Study the drawing (mm; zero at the part's minimum x, y, z) and answer. A direction names the side the tool comes from. Give positions to 0.01 mm unless a question says otherwise; leave off trailing zeros. Order: outer loops, then holes, each group sorted by start corner. A loop starts at its lowest first (then second) coordinate and runs counter-clockwise, first axis right, second up. Notation, with made-up numbers: (-21, 73) - (16, 73) arc R30 cw to (16, 104) - close; hole circle Ø3 at (-25, 48.25). An arc over 180 degrees is marked (long way). Return JSON: item names as keys, results as strings.
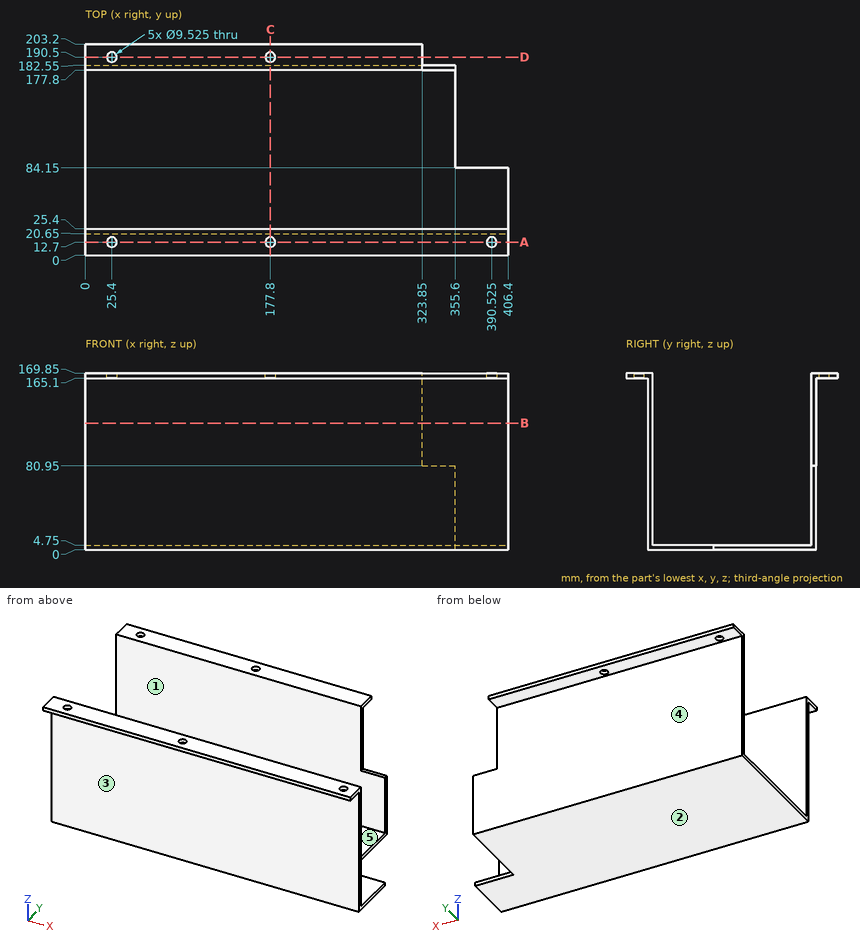
Q1. Given pin 1 (4 mm diameter, centred on x = 268, z = 87.5, fed in from -Y); pin 2 (8.5 mm diameter, centred on x = 25.4, y = 190.5, fed in from -Z); pin 3 (1.4 mm diameter, centred on x = 379.5, z = 1, fed in from +Y); pin 4 (10.5 mm diameter, centred on x = 215.5, y = 10, fed in from -Z), each flat-ended and moving along its own axis, determine where each tip first touches the part or whether it passes through.
Values:
{"pin 1": "stops at y = 20.65", "pin 2": "passes through", "pin 3": "stops at y = 84.15", "pin 4": "stops at z = 165.1"}
Q2. For the marked faces 4 and 5, determine the directions among +Z, -Z, +X, -X, +Y, -Y from which every point of the face is accessible in a straight line to the end or side of a thin tool.
Values:
{"face 4": "-Z, +X, -X, +Y", "face 5": "+Z, +X, -X"}
Q3. A cutting plane is placed at A-A (y = 12.7). Write down the section's boundary in (x, z).
Values:
{"outline": "(0, 165.1) - (20.64, 165.1) - (20.64, 169.85) - (0, 169.85) - close; (30.16, 165.1) - (173.04, 165.1) - (173.04, 169.85) - (30.16, 169.85) - close; (182.56, 165.1) - (385.76, 165.1) - (385.76, 169.85) - (182.56, 169.85) - close; (395.29, 165.1) - (406.4, 165.1) - (406.4, 169.85) - (395.29, 169.85) - close"}
Q4. A cutting plane is placed at D-D (y = 190.5). Write down the section's boundary in (x, z).
Values:
{"outline": "(0, 165.1) - (20.64, 165.1) - (20.64, 169.85) - (0, 169.85) - close; (30.16, 165.1) - (173.04, 165.1) - (173.04, 169.85) - (30.16, 169.85) - close; (182.56, 165.1) - (323.85, 165.1) - (323.85, 169.85) - (182.56, 169.85) - close"}
Q5. Determine the mould class of the marked faces 1, 2 and 3 for opening direction Y: released by +Y, released by -Y, zero draft, split by the parting line, or undercut.
Values:
{"face 1": "undercut", "face 2": "zero draft", "face 3": "released by -Y"}
Q6. Consider L1, parallel to Y at x = 25, z = 168; L2, parallel to X at y = 12, z = 167; L3, parallel to Y at x = 25.4, z = 168.3. Determine where each line is inside the solid, lowest interval first.
Values:
{"L1": "y = 0 to 7.95, 17.45 to 25.4, 177.8 to 185.75, 195.25 to 203.2", "L2": "x = 0 to 20.69, 30.11 to 173.09, 182.51 to 385.81, 395.24 to 406.4", "L3": "y = 0 to 7.94, 17.46 to 25.4, 177.8 to 185.74, 195.26 to 203.2"}
Q7. A cutting plane is placed at C-C (x = 177.8). Write down the section's boundary in (y, z).
Values:
{"outline": "(0, 165.1) - (7.94, 165.1) - (7.94, 169.85) - (0, 169.85) - close; (17.46, 165.1) - (20.65, 165.1) - (20.65, 0) - (182.55, 0) - (182.55, 165.1) - (185.74, 165.1) - (185.74, 169.85) - (177.8, 169.85) - (177.8, 4.75) - (25.4, 4.75) - (25.4, 169.85) - (17.46, 169.85) - close; (195.26, 165.1) - (203.2, 165.1) - (203.2, 169.85) - (195.26, 169.85) - close"}
Q8. A cutting plane is placed at B-B (z = 122). Write down the section's boundary in (x, y).
Values:
{"outline": "(0, 20.65) - (406.4, 20.65) - (406.4, 25.4) - (0, 25.4) - close; (0, 177.8) - (323.85, 177.8) - (323.85, 182.55) - (0, 182.55) - close"}
